For this review, use the dimensioned drawing (mm, ordinates from the lowest corner) and the shaded views. A direction names the side the tool comes from. Coordinates: 2 decimals unless noted, no trailing zeros. Order: outer loops, then holes, each group sorted by start corner. A loop starts at its lowest first (then second) coordinate and runs counter-clockwise, first axis right, second up. Notation, with made-up numbers: (45.5, 0.5) -> (66.5, 0.5) arc R16 cw to (66.5, 9.5) -> close; hole circle Ø4 at (6, -7.5). An arc over 180 degrees is marked (long way). Use one line per item in the form item = value. Start each with the question number.
(1) Wall thickness on line 1 along Z through (x, y) = (65, 6.5); line 2 along Y through (x, z) = (24, 8.5); line 3 along Z through (x, y) = (95, 7.5): over which ranges is each line inside the solid? List them lowest first.
(2) Take a section at B-B (x = 49). State the section outline as (y, z) points, then the cut area to 3 significant figures.
(3) Take a section at A-A (z = 75). State the section outline as (x, y) points.
(4) For the marked faces 1, 2 and 3, list the 3-axis set-ups (+Z, -Z, +X, -X, +Y, -Y) from which the entire face can be reached by the end or side of a thin tool; tool diameter is ignored.
(5) Take a section at C-C (x = 65). State the section outline as (y, z) points.
(6) Take a section at D-D (x = 29). State the section outline as (y, z) points, then the cut area to 3 significant figures.
(7) Insertion check: pin 1 Ø8 at (y, z) = (3, 71) entering from -X; pin 2 Ø10 at (x, z) = (49, 56) entering from +Y; pin 3 Ø1.5 at (x, y) = (103.5, 79.5) entering from +Z. Each pin has a flat end and moves straight along its axis. Give the tip position at first contact, or say it passes through.
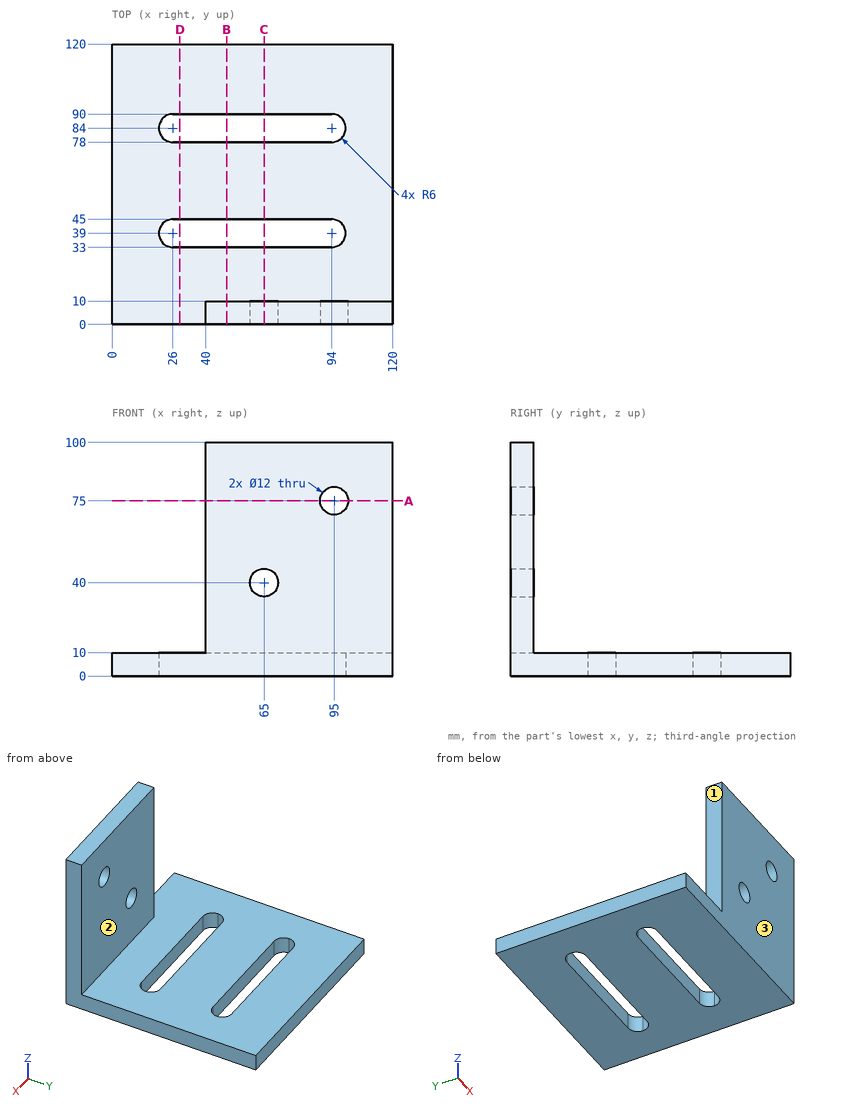
Findings:
q1.line_1 = 0 to 34, 46 to 100
q1.line_2 = 0 to 33.34, 44.66 to 78.34, 89.66 to 120
q1.line_3 = 0 to 69, 81 to 100
q2.outline = (0, 0) -> (33, 0) -> (33, 10) -> (10, 10) -> (10, 100) -> (0, 100) -> close; (45, 0) -> (78, 0) -> (78, 10) -> (45, 10) -> close; (90, 0) -> (120, 0) -> (120, 10) -> (90, 10) -> close
q2.area = 1,860 mm²
q3.outline = (40, 0) -> (89, 0) -> (89, 10) -> (40, 10) -> close; (101, 0) -> (120, 0) -> (120, 10) -> (101, 10) -> close
q4.face_1 = +Z, -X, +Y, -Y
q4.face_2 = +Z, +X, -X, +Y
q4.face_3 = +Z, -Z, +X, -X, -Y
q5.outline = (0, 0) -> (33, 0) -> (33, 10) -> (10, 10) -> (10, 34) -> (0, 34) -> close; (0, 46) -> (10, 46) -> (10, 100) -> (0, 100) -> close; (45, 0) -> (78, 0) -> (78, 10) -> (45, 10) -> close; (90, 0) -> (120, 0) -> (120, 10) -> (90, 10) -> close
q6.outline = (0, 0) -> (33, 0) -> (33, 10) -> (0, 10) -> close; (45, 0) -> (78, 0) -> (78, 10) -> (45, 10) -> close; (90, 0) -> (120, 0) -> (120, 10) -> (90, 10) -> close
q6.area = 960 mm²
q7.pin_1 = 40
q7.pin_2 = 10
q7.pin_3 = 10
